Job drawing, mm, ordinate dimensions from the low corner. One solid piece. A direction names the side the tool comes from. Coordinates: 2 decimals unless noted, no trailing zeros. Write each loop counter-clockwise with the first axis right and the second up, starting at its lowest first coordinate (ties: lowest second). Pieces come first, ordered by that corner, then holes. Notation, with made-up numbers: (83.25, -26.75) - (103.25, -26.75) arc R29 cw to (103.25, -4.75) - close; hole circle Ø11 at (48, 15.5). An arc over 180 degrees is marked (long way). Put each result on its own line as item: value. Start each with the question number.
1. Saw through at A-A, the plane y = 17.5. Write the cut outline in (x, z).
2. Drill centre lines: L1, parallel to X at y = 25, z = 5.5; L2, parallel to X at y = 24.5, z = 26; L3, parallel to Z at x = 92, y = 18. Where is each one in solid material? Low to high. Write a range as from..to.
3. Saw through at C-C, the plane x = 53. Write the cut outline in (y, z), plus the area to 3 significant figures.
4. Saw through at D-D, the plane z = 27. Write the cut outline in (x, y).
5. Which spindle directions (+Z, -Z, +X, -X, +Y, -Y) get a long thin tool onto all of the face, cutting with end or side? Do the marked faces 1 and 2. Say none if no direction does.
6. Drop flat-ended pins along their axis: P1, Ø6, axis at x = 42, z = 18.5, coming from the -Y side; P2, Ø4, axis at x = 84, y = 26.5, coming from the +Z side; P3, Ø6, axis at x = 88.5, y = 16, coming from the -Z side. Give the stop position or say it passes through.
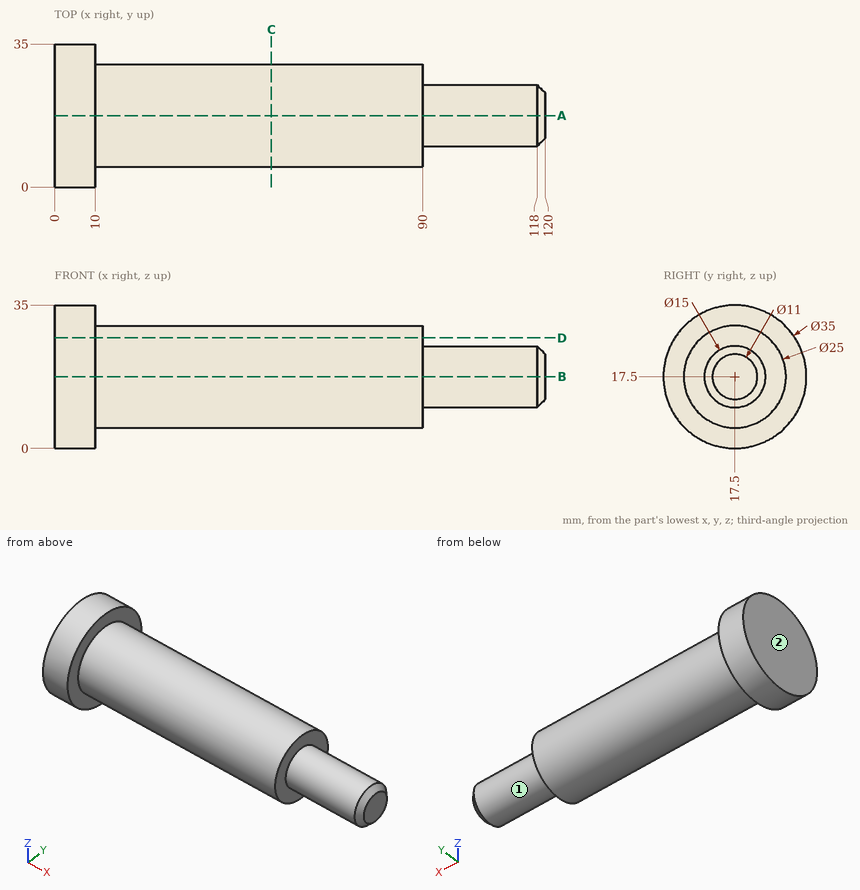
Final values:
1. outline: (0, 0) - (10, 0) - (10, 5) - (90, 5) - (90, 10) - (118, 10) - (120, 12) - (120, 23) - (118, 25) - (90, 25) - (90, 30) - (10, 30) - (10, 35) - (0, 35) - close
2. L1: x = 0..10
2. L2: x = 0..90
2. L3: z = 10.02..24.98
3. outline: circle Ø25 at (17.5, 17.5)
3. area: 491 mm²
4. outline: (0, 2.8) - (10, 2.8) - (10, 9.38) - (90, 9.38) - (90, 25.62) - (10, 25.62) - (10, 32.2) - (0, 32.2) - close
5. face 1: +X
5. face 2: +Z, -Z, -X, +Y, -Y
6. P1: stops at y = 5
6. P2: stops at z = 27.86
6. P3: stops at z = 5
